Model file for the job. Use its own axes, mm. A direction names the side the tool comes from. Round coordinates to 2 decimals unless told otherwise and drop trailing zeros. Order: outer loops, then holes, each group sorted by start corner. A loop starts at its lowest first (then second) coordinate and runs counter-clockwise, first axis right, second up. Notation, with made-up numbers: (45.25, -25) - (90.25, -25) arc R13 cw to (90.25, -10) - close; hole circle Ø7 at (27.25, 70). An arc over 180 degrees is marked (long way). Put each result on its own line as item: value. Start each with the question number.
Item 1: Mould opens along Z. For faces 3 (the face through (-0.826, -54.79, -19.554)), 4 (the face through (2.927, -54.79, 19.317)), 5 (the face through (23.846, -19.72, -7.509)), 6 (the face through (0, -70, 14)) say: pulls with the +Z half, pulls with the -Z half, needs draft (parallel to the pull), parting line crosses it, or undercut.
Item 2: Which spindle directions (+Z, -Z, +X, -X, +Y, -Y) get a long thin tool onto all of the face, cutting with end or side? Do faces 1 (the face through (0, -70, -13)), 2 (the face through (0, -40, 0)). Say none if no direction does.
Item 3: Probe probe 1 along Z at (x, y) = (0.5, 0.5); probe 2 along Z at (x, y) = (5, 12); probe 3 along Y at (x, z) = (-16, 17). List the from-to ranges inside material, lowest first.
Item 4: Saw through at B-B on z = 11. List the corners of the cut face in (x, y), plus the area to 3 significant figures.
Item 5: Saw through at A-A on x = 0. List the corners of the cut face in (y, z), plus the area to 3 significant figures.
Item 6: Saw through at C-C on y = -55. List the corners of the cut face in (x, z), plus the area to 3 significant figures.
Item 7: Saw through at D-D on y = -8.5. List the corners of the cut face in (x, z).
Item 8: Pin check, flat tips, straight feed: pin 1 Ø1.5 at (y, z) = (12.5, -4.5) entering from -X; pin 2 Ø6 at (x, y) = (8.5, -44.5) entering from +Z; pin 3 Ø5 at (x, y) = (8, -12) entering from -Z. Stop position of each tip, or through.
Autodesk Inventor part; units mm, degrees
ref_plane "YZ Plane" through (0, 0, 0) normal (1, 0, 0) x (0, 1, 0)
ref_plane "XZ Plane" through (0, 0, 0) normal (0, 1, 0) x (-1, 0, 0)
ref_plane "XY Plane" through (0, 0, 0) normal (0, 0, 1) x (1, 0, 0)
sketch "Sketch1" plane through (0, 0, 0) normal (0, 1, 0) x (-1, 0, 0)
  arc A0 (0, -25) -> (0, 25) centre (0, 0) ccw
  line L0 (0, 25) -> (0, -25)
  dimension "d0" = 50
revolve "Revolution1" add sketch "Sketch1" angle 180 about axis through (0, 0, 25) along (0, 0, -1)
sketch "Sketch2" plane through (0, 0, 0) normal (0, -1, 0) x (1, 0, 0)
  circle A0 centre (0, 0) radius 25
extrude "Extrusion1" add sketch "Sketch2" along normal blind 40
sketch "Sketch3" plane through (0, -40, 0) normal (0, -1, 0) x (1, 0, 0)
  circle A0 centre (0, 13.6892) radius 6.3431
  circle A1 centre (0, -13.2647) radius 6.3431
  point P0 (0, 0)
extrude "Extrusion2" add sketch "Sketch3" along normal blind 30
properties part number "yellow led now"
Results found:
1. face 3: undercut
1. face 4: undercut
1. face 5: parting line crosses it
1. face 6: needs draft
2. face 1: +Z, -Z, +X, -X, -Y
2. face 2: -Y
3. probe 1: z = -24.99 to 24.99
3. probe 2: z = -21.35 to 21.35
3. probe 3: y = -40 to 8.94
4. outline: (-22.45, -40) - (-5.74, -40) - (-5.74, -70) - (5.74, -70) - (5.74, -40) - (22.45, -40) - (22.45, 0) arc R22.45 ccw to (-22.45, 0) - close
4. area: 2,930 mm²
5. outline: (-70, -19.61) - (-40, -19.61) - (-40, -25) - (0, -25) arc R25 ccw to (0, 25) - (-40, 25) - (-40, 20.03) - (-70, 20.03) - (-70, 7.35) - (-40, 7.35) - (-40, -6.92) - (-70, -6.92) - close
5. area: 3,740 mm²
6. outline: circle Ø12.69 at (0, -13.26); circle Ø12.69 at (0, 13.69)
6. area: 253 mm²
7. outline: circle Ø50 at (0, 0)
8. pin 1: stops at x = -21.63
8. pin 2: stops at z = 16.85
8. pin 3: stops at z = -24.39
